Part model, mm, in its own coordinate system. A direction names the side the tool comes from. Give positions to 0.01 mm unless a question says otherwise; leave off trailing zeros. Write each loop counter-clockwise with the first axis right and the second up, starting at its lowest first coordinate (ties: lowest second). Pieces come first, ordered by that corner, then holes.
Autodesk Inventor part; units mm, degrees
ref_plane "YZ Plane" through (0, 0, 0) normal (1, 0, 0) x (0, 1, 0)
ref_plane "XZ Plane" through (0, 0, 0) normal (0, 1, 0) x (-1, 0, 0)
ref_plane "XY Plane" through (0, 0, 0) normal (0, 0, 1) x (1, 0, 0)
sketch "Sketch1" plane through (0, 0, 0) normal (0, 1, 0) x (-1, 0, 0)
  line L0 (0, 0) -> (-37, 0)
  line L1 (-37, 0) -> (-37, -37)
  line L2 (-37, -37) -> (0, -37)
  line L3 (0, -37) -> (0, 0)
  circle A0 centre (-5.5, -5.5) radius 2
  circle A1 centre (-5.5, -31.5) radius 2
  circle A2 centre (-31.5, -5.5) radius 2
  circle A3 centre (-31.5, -31.5) radius 2
  circle A4 centre (-18.5, -18.5) radius 12
  dimension "d10" = 24
extrude "Extrusion1" add sketch "Sketch1" along normal blind 3
sketch "Sketch2" plane through (0, 3, 0) normal (0, 1, 0) x (1, 0, 0)
  circle A0 centre (18.5, 18.5) radius 12
  circle A1 centre (31.5, 31.5) radius 2
  circle A2 centre (31.5, 5.5) radius 2
  circle A3 centre (5.5, 31.5) radius 2
  circle A4 centre (5.5, 5.5) radius 2
  line L0 (0, 0) -> (37, 0)
  line L1 (37, 37) -> (0, 37)
  line L2 (0, 37) -> (0, 0)
  line L3 (-3, -3) -> (37, -3)
  line L4 (37, 40) -> (-3, 40)
  line L5 (-3, 40) -> (-3, -3)
  line L6 (37, -3) -> (37, 0)
  line L7 (37, 37) -> (37, 40)
  dimension "d13" = 3
extrude "Extrusion2" add sketch "Sketch2" along normal blind 60 and the other way blind 3 contours L0 L6 L3 L5 L4 L7 L1 L2
sketch "Sketch4" plane through (0, 63, 0) normal (0, 1, 0) x (1, 0, 0)
  circle A0 centre (18.5, 18.5) radius 12
  circle A1 centre (31.5, 31.5) radius 2
  circle A2 centre (31.5, 5.5) radius 2
  circle A3 centre (5.5, 31.5) radius 2
  circle A4 centre (5.5, 5.5) radius 2
  line L0 (0, 0) -> (37, 0)
  line L1 (37, 0) -> (37, 37)
  line L2 (37, 37) -> (0, 37)
  line L3 (0, 37) -> (0, 0)
  line L4 (37, 0) -> (0, 0)
  line L5 (0, 0) -> (0, 37)
  line L6 (0, 37) -> (37, 37)
  line L7 (37, 37) -> (37, 40)
  line L8 (37, 40) -> (-3, 40)
  line L9 (-3, 40) -> (-3, -3)
  line L10 (-3, -3) -> (37, -3)
  line L11 (37, -3) -> (37, 0)
extrude "Extrusion3" add sketch "Sketch4" along normal blind 3
sketch "Sketch5" plane through (0, 66, 0) normal (0, 1, 0) x (1, 0, 0)
  arc A0 (29.4087, 13.5) -> (29.4087, 23.5) centre (18.5, 18.5) ccw
  circle A1 centre (5.5, 5.5) radius 2
  circle A2 centre (5.5, 31.5) radius 2
  circle A3 centre (31.5, 5.5) radius 2
  circle A4 centre (31.5, 31.5) radius 2
  line L0 (37, 13.5) -> (37, 23.5)
  line L1 (37, 40) -> (-3, 40)
  line L2 (-3, 40) -> (-3, -3)
  line L3 (-3, -3) -> (37, -3)
  arc A5 (29.4087, 13.5) -> (29.4087, 23.5) centre (18.5, 18.5) ccw
  line L4 (37, 23.5) -> (37, 13.5)
  line L5 (29.4087, 23.5) -> (37, 23.5)
  line L6 (29.4087, 13.5) -> (37, 13.5)
  point P0 (0, 0)
extrude "Extrusion4" cut sketch "Sketch5" against normal up to surface (66 mm away) contours A0 L5 L0 L6
fillet "Fillet1" radius 4 8 edges at (29.4087, 64.5, -13.5) (37, 64.5, -13.5) (37, 64.5, -23.5) (29.4087, 64.5, -23.5) (37, 1.5, -13.5) (29.4087, 1.5, -13.5) (37, 1.5, -23.5) (29.4087, 1.5, -23.5)
sketch "Sketch7" plane through (37, 0, -40) normal (0, 0, -1) x (-1, 0, 0)
  line L0 (40, 66) -> (40, 0)
  line L1 (0, 66) -> (40, 66)
  line L2 (0, 66) -> (0, 0)
  line L3 (40, 0) -> (0, 0)
  line L4 (30, 56) -> (30, 10)
  line L5 (30, 10) -> (10, 10)
  line L6 (10, 10) -> (10, 56)
  line L7 (10, 56) -> (30, 56)
  point P0 (37, 0)
  dimension "d26" = 10
extrude "Extrusion5" cut sketch "Sketch7" against normal up to surface (43 mm away) contours L4 L5 L6 L7
sketch "Sketch8" plane through (-3, 0, -40) normal (-1, 0, 0) x (0, 0, 1)
  line L0 (43, 66) -> (43, 0)
  line L1 (0, 66) -> (43, 66)
  line L2 (0, 66) -> (0, 0)
  line L3 (43, 0) -> (0, 0)
  line L4 (33, 56) -> (33, 10)
  line L5 (33, 10) -> (10, 10)
  line L6 (10, 10) -> (10, 56)
  line L7 (10, 56) -> (33, 56)
  point P0 (40, 0)
  dimension "d29" = 10
extrude "Extrusion6" cut sketch "Sketch8" against normal blind 3 contours L4 L5 L6 L7
sketch "Sketch9" plane through (-3, 0, -40) normal (-1, 0, 0) x (0, 0, 1)
  line L0 (10, 56) -> (33, 56)
  line L1 (33, 56) -> (33, 10)
  line L2 (33, 10) -> (10, 10)
  line L3 (10, 10) -> (10, 56)
  line L4 (0, 66) -> (43, 66)
  line L5 (43, 0) -> (0, 0)
  line L6 (0, 66) -> (43, 66)
  circle A0 centre (50.075, 8.87) radius 2
  circle A1 centre (-15.965, 12.045) radius 2
  circle A2 centre (50.075, 57.13) radius 2
  circle A3 centre (-15.965, 53.955) radius 2
  arc A4 (50.075, 3.87) -> (50.075, 13.87) centre (50.075, 8.87) ccw
  arc A5 (50.075, 52.13) -> (50.075, 62.13) centre (50.075, 57.13) ccw
  arc A6 (-15.965, 17.045) -> (-15.965, 7.045) centre (-15.965, 12.045) ccw
  arc A7 (-15.965, 58.955) -> (-15.965, 48.955) centre (-15.965, 53.955) ccw
  line L7 (50.075, 3.87) -> (43, 3.87)
  line L8 (50.075, 13.87) -> (43, 13.87)
  line L9 (50.075, 62.13) -> (43, 62.13)
  line L10 (50.075, 52.13) -> (43, 52.13)
  line L11 (-15.965, 7.045) -> (0, 7.045)
  line L12 (-15.965, 17.045) -> (0, 17.045)
  line L13 (-15.965, 48.955) -> (0, 48.955)
  line L14 (0, 56) -> (0, 10)
  line L15 (-15.965, 58.955) -> (0, 58.955)
  line L16 (0, 66) -> (0, 0)
  line L17 (0, 58.955) -> (0, 48.955)
  line L18 (0, 17.045) -> (0, 7.045)
  line L19 (43, 62.13) -> (43, 52.13)
  line L20 (43, 13.87) -> (43, 3.87)
  point P0 (40, 0)
  dimension "d53" = 10
extrude "Extrusion7" add sketch "Sketch9" against normal blind 3 contours L7 L20 L8 A4 | L10 L19 L9 A5 | L12 L14 L16 L11 A6 | L13 A7 L15 L16 L14
properties part number "14HM11 Chassis"
1) Pin check, flat tips, straight feed: pin 1 Ø12 at (x, y) = (18.5, 34) entering from -Z; pin 2 Ø8 at (y, z) = (20.5, -5.5) entering from +X; pin 3 Ø2.5 at (x, z) = (-1.5, -15) entering from -Y; pin 4 Ø20 at (x, y) = (11, 40.5) entering from +Z. Stop position of each tip, or through.
Answers follow:
pin 1: passes through
pin 2: stops at x = 0
pin 3: stops at y = 0
pin 4: stops at z = 3
2) Saw through at B-B, the plane z = 5. Write the cut outline in (x, y).
Answers follow:
outline: (-3, 3.87) - (0, 3.87) - (0, 13.87) - (-3, 13.87) - close; (-3, 52.13) - (0, 52.13) - (0, 62.13) - (-3, 62.13) - close
3) Saw through at A-A, the plane z = -5.5. Write the cut outline in (x, y).
Answers follow:
outline: (-3, 0) - (3.5, 0) - (3.5, 3) - (0, 3) - (0, 63) - (3.5, 63) - (3.5, 66) - (-3, 66) - close; (7.5, 0) - (29.5, 0) - (29.5, 3) - (7.5, 3) - close; (7.5, 63) - (29.5, 63) - (29.5, 66) - (7.5, 66) - close; (33.5, 0) - (37, 0) - (37, 3) - (33.5, 3) - close; (33.5, 63) - (37, 63) - (37, 66) - (33.5, 66) - close
4) 3-axis set-ups, long thin cutter, end or side, ignore diameter. For faces 4 (the face through (6, 63, -19)), 5 (the face through (7, 33, 1)), 6 (the face through (29.83, 64.48, -13.02)), 7 (the face through (0, 8.9, 7.6)), 8 (the face through (35.859, 1.479, -24.703)): which of +Z, -Z, +X, -X, +Y, -Y reach the whole face in a straight line?
Answers follow:
face 4: +X
face 5: +Z, -Z
face 6: +Y, -Y
face 7: +Z, +X, +Y, -Y
face 8: +X, +Y, -Y
5) Wall check: L1, parallel to Z at x = 31.5, y = 64.6; L2, parallel to Z at x = 31.5, y = 35; L3, parallel to Z at x = -0.5, y = 27.5. Give the ranges that are in metal, low to high.
Answers follow:
L1: z = -40 to -33.5, -29.5 to -23.51, -13.49 to -7.5, -3.5 to 3
L2: z = -40 to -37, 0 to 3
L3: z = -40 to -30, -7 to 3
6) Two-plate mould, pull along Z, no slides. Class faces 1 (the face through (-1.521, 54.065, -60.964)), 2 (the face through (0, 54, -51)), 3 (the face through (3.9, 64.5, -6.7)): +Z half, -Z half, draft (parallel to the pull), parting line (faces both ways), or undercut.
Answers follow:
face 1: -Z half
face 2: draft
face 3: undercut
7) Saw through at D-D, the plane y = 19. Write the cut outline in (x, z), then the cut area to 3 significant figures.
Answers follow:
outline: (-3, -40) - (7, -40) - (7, -37) - (0, -37) - (0, -30) - (-3, -30) - close; (-3, -7) - (0, -7) - (0, 0) - (7, 0) - (7, 3) - (-3, 3) - close; (27, -40) - (37, -40) - (37, -37) - (27, -37) - close; (27, 0) - (37, 0) - (37, 3) - (27, 3) - close
area: 162 mm2
8) Saw through at C-C, the plane x = 18.5. Write the cut outline in (y, z).
Answers follow:
outline: (0, -40) - (10, -40) - (10, -37) - (3, -37) - (3, -30.5) - (0, -30.5) - close; (0, -6.5) - (3, -6.5) - (3, 0) - (10, 0) - (10, 3) - (0, 3) - close; (56, -40) - (66, -40) - (66, -30.5) - (63, -30.5) - (63, -37) - (56, -37) - close; (56, 0) - (63, 0) - (63, -6.5) - (66, -6.5) - (66, 3) - (56, 3) - close
